from build123d import *

# Parameters (mm, degrees)
BOSS_EXTRUDE1_DEPTH = 4
CUT_EXTRUDE1_DEPTH  = 10
SKETCH6_R           = 40.091527734
CUT_EXTRUDE2_DEPTH  = 4
FILLET1_START       = -1
FILLET1_DEPTH       = 6


with BuildPart() as part:
    # Sketch1 → Boss-Extrude1 (new body)
    with BuildSketch(Plane.XY):
        with BuildLine():
            Line((76.333328469, 66.289722012), (74.505251863, 66.289722012))
            ThreePointArc((74.505251863, 66.289722012), (71.161019545, 65.339696261), (68.815702909, 62.773389851))
            ThreePointArc((68.815702909, 62.773389851), (60.349327785, 48.779313667), (49.750676494, 36.322096209))
            ThreePointArc((49.750676494, 36.322096209), (34.635353478, 21.965885228), (23.967617679, 4.055742947))
            ThreePointArc((23.967617679, 4.055742947), (14.404733147, -9.267078846), (-1.356711824, -13.797331986))
            ThreePointArc((-1.356711824, -13.797331986), (-15.492367955, -8.455246222), (-23.967617153, 4.055741173))
            ThreePointArc((-23.967617153, 4.055741173), (-31.555286979, 21.388261286), (-43.172925895, 36.322097125))
            ThreePointArc((-43.172925895, 36.322097125), (-52.235366406, 48.931803578), (-59.274045863, 62.773390061))
            ThreePointArc((-59.274045863, 62.773390061), (-61.619362494, 65.339696323), (-64.963594711, 66.289722012))
            Line((-64.963594711, 66.289722012), (-76.333336807, 66.289722012))
            ThreePointArc((-76.333336807, 66.289722012), (-103.321243377, 55.110962932), (-114.5, 28.123055345))
            Line((-114.5, 28.123055345), (-114.5, -133.710277988))
            Line((-114.5, -133.710277988), (114.5, -133.710277988))
            Line((114.5, -133.710277988), (114.5, 28.123055345))
            ThreePointArc((114.5, 28.123055345), (103.321240429, 55.11096588), (76.333328469, 66.289722012))
        make_face()
    extrude(amount=BOSS_EXTRUDE1_DEPTH)

    # Sketch2 → Cut-Extrude1 (cut)
    with BuildSketch(Plane.XY.offset(4)):
        with BuildLine():
            Line((-95.500001569, -56.710277988), (-95.500001569, -121.710277988))
            ThreePointArc((-95.500001569, -121.710277988), (-99.500001569, -125.710277988), (-103.500001569, -121.710277988))
            Line((-103.500001569, -121.710277988), (-103.500001569, -56.710277988))
            ThreePointArc((-103.500001569, -56.710277988), (-99.500001569, -52.710277988), (-95.500001569, -56.710277988))
        make_face()
        with BuildLine():
            Line((95.500001569, -56.710277988), (95.500001569, -121.710277988))
            ThreePointArc((95.500001569, -121.710277988), (99.500001569, -125.710277988), (103.500001569, -121.710277988))
            Line((103.500001569, -121.710277988), (103.500001569, -56.710277988))
            ThreePointArc((103.500001569, -56.710277988), (99.500001569, -52.710277988), (95.500001569, -56.710277988))
        make_face()
    extrude(amount=-CUT_EXTRUDE1_DEPTH, mode=Mode.SUBTRACT)

    # Sketch6 → Cut-Extrude2 (cut)
    with BuildSketch(Plane.XY.offset(4)):
        with Locations((-1.216e-06, 11.16582753)):
            Circle(SKETCH6_R)
    extrude(amount=-CUT_EXTRUDE2_DEPTH, mode=Mode.SUBTRACT)

    # Fillet1: read off the stored shape, not the designer's step
    # Fillet1 outline → Fillet1 (cut)
    with BuildSketch(Plane.XY.offset(FILLET1_START)):
        with BuildLine():
            ThreePointArc((-43.172925895, 36.322097125), (-46.764931779, 40.845410754), (-50.094550883, 45.56521044))
            ThreePointArc((-50.094550883, 45.56521044), (-42.536890866, 29.36311637), (-40.088563254, 11.653464507))
            ThreePointArc((-40.088563254, 11.653464507), (-39.059263062, 20.20489054), (-36.227182581, 28.339118606))
            ThreePointArc((-36.227182581, 28.339118606), (-39.561558424, 32.4511088), (-43.172925895, 36.322097125))
        make_face()
        with BuildLine():
            ThreePointArc((37.500310301, 25.345292688), (39.69442098, 16.794632252), (39.964034241, 7.971071505))
            ThreePointArc((39.964034241, 7.971071505), (43.057284902, 22.767959834), (49.750676494, 36.322096209))
            ThreePointArc((49.750676494, 36.322096209), (43.328961969, 31.16463037), (37.500310301, 25.345292688))
        make_face()
    extrude(amount=FILLET1_DEPTH, mode=Mode.SUBTRACT)


solid = part.part
The listing builds one solid part. Answer for the finished solid, in the listing's coordinates (mm). A direction names the side the tool comes from. Round coordinates to 2 decimals unless told otherwise and drop trailing zeros. Write each loop counter-clockwise with the first axis right and the second up, starting at its lowest first coordinate (ties: lowest second). Pieces come first, ordered by that corner, then holes. Notation, with made-up numbers: M 36.25,7.5 L 68.25,7.5 A22 ccw 68.25,14.5 Z; hole C -26.75,-0.75 d11. An arc over 180 degrees is marked long. Write each question's results on one line, items separated by ' | '. Start each with the question number.
(1) The part is cut by section A-A, the plane y = 51.5. Write down the section's boundary in (x, z).
(2) This flat-tipped pin is pushed along its axis until it touches: P1, Ø1, axis at x = -77, z = 2, coming from the +Y side. Where does it stop, or does it pass through?
(3) Find the intervals of material crossed by line 1 (X direction, y = -120, z = 1.2); line 2 (X direction, y = -54, z = 1.8); line 3 (X direction, y = 29, z = 2.35), in increasing order.
(4) The part is cut by section C-C, the plane x = -8. Write down the section's boundary in (y, z).
(5) The part is cut by section B-B, the plane z = 1.3. Write down the section's boundary in (x, y).
(6) Determine the mould class of faces 3 (the cylindrical face through (-42.608, 29.604, 1.972)), 4 (the cylindrical face through (103.62, 54.81, 1.97)), 5 (the flat face through (-2, -32, 0)) for opening direction X: +X half, -X half, draft (parallel to the pull), parting line (faces both ways), or undercut.
(7) The part is cut by section D-D, the plane x = 17.5. Write down the section's boundary in (y, z).
(8) For faces 1 (the flat face through (-2, -32, 4)), 2 (the cylindrical face through (-55.033, 53.828, 1.972)), determine the directions among +Z, -Z, +X, -X, +Y, -Y from which every point of the face is accessible in a straight line to the end or side of a thin tool.
Worked answers:
1) outline: M -106.5,0 L -53.75,0 L -53.75,4 L -106.5,4 Z; M 62.24,0 L 106.5,0 L 106.5,4 L 62.24,4 Z
2) P1: stops at y = 66.29
3) line 1: x = -114.5 to -103.5, -95.5 to 95.5, 103.5 to 114.5 | line 2: x = -114.5 to -102.44, -96.56 to 96.56, 102.44 to 114.5 | line 3: x = -114.49 to -42.43, 45.61 to 114.49
4) outline: M -133.71,0 L -28.12,0 L -28.12,4 L -133.71,4 Z
5) outline: M -114.5,-133.71 L 114.5,-133.71 L 114.5,28.12 A38.17 ccw 76.33,66.29 L 74.51,66.29 A6.36 ccw 68.82,62.77 A101.78 cw 49.75,36.32 A60 ccw 39.96,7.97 A40.09 cw -40.09,11.65 A60 ccw -50.09,45.57 A101.78 cw -59.27,62.77 A6.36 ccw -64.96,66.29 L -76.33,66.29 A38.17 ccw -114.5,28.12 Z; hole M -103.5,-121.71 A4 ccw -95.5,-121.71 L -95.5,-56.71 A4 ccw -103.5,-56.71 Z; hole M 95.5,-121.71 A4 ccw 103.5,-121.71 L 103.5,-56.71 A4 ccw 95.5,-56.71 Z
6) face 3: undercut | face 4: +X half | face 5: draft
7) outline: M -133.71,0 L -24.9,0 L -24.9,4 L -133.71,4 Z
8) face 1: +Z, +X, -X, +Y, -Y | face 2: +Z, -Z, +Y
